from build123d import *

# Parameters (mm, degrees)
SKIZZE2_W                       = 56.2
SKIZZE2_H                       = 56.2
SKIZZE2_W_2                     = 42.2
SKIZZE2_H_2                     = 42.2
AUFSATZ_LINEAR_AUSTRAGEN1_DEPTH = 10
SKIZZE3_W                       = 10
SKIZZE3_H                       = 20
AUFSATZ_LINEAR_AUSTRAGEN2_DEPTH = 20
SKIZZE4_R                       = 2.5
SCHNITT_LINEAR_AUSTRAGEN1_DEPTH = 27
KREISMUSTER1_COUNT              = 3
KREISMUSTER2_COUNT              = 3
VERRUNDUNG1_R                   = 10
VERRUNDUNG2_R                   = 10
VERRUNDUNG3_R                   = 10
VERRUNDUNG4_R                   = 5


with BuildPart() as part:
    # Skizze2 → Aufsatz-Linear austragen1 (new body)
    with BuildSketch(Plane.XY):
        with Locations((21.1, 21.1)):
            Rectangle(SKIZZE2_W, SKIZZE2_H)
        with Locations((21.1, 21.1)):
            Rectangle(SKIZZE2_W_2, SKIZZE2_H_2, mode=Mode.SUBTRACT)
    extrude(amount=AUFSATZ_LINEAR_AUSTRAGEN1_DEPTH)

    # Skizze3 → Aufsatz-Linear austragen2 (add)
    with BuildSketch(Plane(origin=(49.2, 0, 0), x_dir=(0, 0, -1), z_dir=(1, 0, 0))):
        with Locations((-5, 21.1)):
            Rectangle(SKIZZE3_W, SKIZZE3_H)
    aufsatz_linear_austragen2 = extrude(amount=AUFSATZ_LINEAR_AUSTRAGEN2_DEPTH)

    # Skizze4 → Schnitt-Linear austragen1 (cut)
    with BuildSketch(Plane.XY.offset(10)):
        with Locations((59.7, 21.1)):
            Circle(SKIZZE4_R)
    schnitt_linear_austragen1 = extrude(amount=-SCHNITT_LINEAR_AUSTRAGEN1_DEPTH, mode=Mode.SUBTRACT)

    # Kreismuster1: Aufsatz-Linear austragen2 ×3 about axis
    kreismuster1_axis = Axis((21.1, 21.1, 0), (0, 0, 1))
    for i in range(1, KREISMUSTER1_COUNT):
        add(aufsatz_linear_austragen2.rotate(kreismuster1_axis, i * 360 / KREISMUSTER1_COUNT))

    # Kreismuster2: Schnitt-Linear austragen1 ×3 about axis
    kreismuster2_axis = Axis((21.1, 21.1, 0), (0, 0, 1))
    for i in range(1, KREISMUSTER2_COUNT):
        add(schnitt_linear_austragen1.rotate(kreismuster2_axis, i * 360 / KREISMUSTER2_COUNT), mode=Mode.SUBTRACT)

    # Verrundung1
    # the kernel refuses this fillet: 10 mm, written as the material it adds along each edge
    with BuildSketch(Plane(origin=(13.570627693, 49.2, 10), x_dir=(0.866025403783509, 0.5000000000016102, 0), z_dir=(0, 0, -1))) as verrundung1_piece_1:
        with BuildLine():
            CenterArc((11.022527997, -5.183145878), VERRUNDUNG1_R, 120, 28.780734866)
            Line((6.022527997, 3.47710816), (0, 0))
            Line((0, 0), (2.470627693, 0))
        make_face()
    extrude(amount=10)

    # Verrundung2
    # the kernel refuses this fillet: 10 mm, written as the material it takes off along each edge
    with BuildSketch(Plane(origin=(-7, 49.2, -6.36420772), x_dir=(0, -1, 0), z_dir=(0, 0, 1))) as verrundung2_piece_1:
        with BuildLine():
            CenterArc((2.545683088, 10), VERRUNDUNG2_R, 255.251993066, 14.748006934)
            Line((0, 0.329452052), (-0.050913662, 0.136041093))
            ThreePointArc((-0.050913662, 0.136041093), (-0.2, 0.164726026), (-0.2, 0))
            Line((-0.2, 0), (0, -0.2))
            Line((0, -0.2), (2.545683088, -0.2))
            Line((2.545683088, -0.2), (2.545683088, 0))
        make_face()
    extrude(amount=22.72841544, mode=Mode.SUBTRACT)

    # Verrundung3
    # the kernel refuses this fillet: 10 mm, written as the material it adds along each edge
    with BuildSketch(Plane(origin=(13.570627693, -7, 0), x_dir=(1, 0, 0), z_dir=(0, 0, 1))) as verrundung3_piece_1:
        with BuildLine():
            CenterArc((6.95421632, -10), VERRUNDUNG3_R, 90, 28.780734866)
            Line((2.139626345, -1.235313846), (0, 0))
            Line((0, 0), (6.95421632, 0))
        make_face()
    extrude(amount=10)
    # the kernel refuses this fillet: 10 mm, written as the material it takes off along each edge
    with BuildSketch(Plane(origin=(-7, -7, -6.36420772), x_dir=(1, 0, 0), z_dir=(0, 0, 1))) as verrundung3_2_piece_1:
        with BuildLine():
            CenterArc((10, 2.545683088), VERRUNDUNG3_R, 180, 14.748006934)
            Line((0, 2.545683088), (0, 0))
            Line((0, 0), (0.329452052, 0))
        make_face()
    extrude(amount=22.72841544, mode=Mode.SUBTRACT)

    # Verrundung4
    verrundung4_edges = [part.edges().sort_by_distance(p)[0] for p in [
        (49.2, 11.1, 5),
        (49.2, 31.1, 5),
    ]]
    fillet(verrundung4_edges, radius=VERRUNDUNG4_R)


solid = part.part
The model under review builds one solid part; all positions refer to its coordinate system, in mm. A direction names the side the tool comes from. Round coordinates to 2 decimals unless told otherwise and drop trailing zeros. Write each loop counter-clockwise with the first axis right and the second up, starting at its lowest first coordinate (ties: lowest second). Pieces come first, ordered by that corner, then holes. Notation, with made-up numbers: M -22,-14 L 10,-14 A28 cw 10,16 Z; hole C 56,32.25 d2. An arc over 180 degrees is marked long. Use a Markdown table: item, result. Add a question column.
Q1. Insertion check: pin 1 (5 mm diameter, centred on x = 37.5, z = 7.5, fed in from -Y); pin 2 (3 mm diameter, centred on x = 14, z = 2.5, fed in from +Y); pin 3 (4 mm diameter, centred on y = -7, z = 1.5, fed in from +X). Each pin has a flat end and moves straight along its axis. Give the tip position at first contact, or say it passes through.
Q2. To check wall thickness, follow line 1 (X direction, y = 17, z = 9.25); line 2 (Y direction, x = 59.7, z = 7.25); line 3 (Y direction, x = 22.5, z = 1.5). State the ranges of each line that lie inside material, in increasing order.
Q3. We need section A-A, the plane y = 21.1. State the section outline as (x, z) points, plus the area to 3 significant figures.
Q4. We need section D-D, the plane z = 1.25. Count the separate pieces of the cut face and the enclosed holes in it, plus the area to 3 significant figures.
Q5. We need section B-B, the plane x = 33. State the section outline as (y, z) points, plus the area to 3 significant figures.
Q6. We need section C-C, the plane y = 8.5. State the section outline as (x, z) points, plus the area to 3 significant figures.
Q7. The part is to be moulded in two halves that separate along Y. For faces 5 (the face through (-9.106, 53.418, 5.07)), 6 (the face through (-1, 18, 10)), 7 (the face through (62, 11.1, 5)), say which applies: pulls with the +Y half, pulls with the -Y half, needs draft (parallel to the pull), parting line crosses it, or undercut.
Q8. Machinability: for faces 1 (the face through (42.2, 21, 5)), 2 (the face through (49.2, 43, 5)), 3 (the face through (35, -7, 5)), 4 (the face through (-6.92, -5.72, 4.93)), which of the approach directions +Z, -Z, +X, -X, +Y, -Y give a long, thin tool a straight path to every point of the face, cutting with its end or side? Answer none if there is none.
Findings below:
| question | item | result |
|---|---|---|
| 1 | pin 1 | stops at y = -7 |
| 1 | pin 2 | stops at y = 56 |
| 1 | pin 3 | stops at x = 49.2 |
| 2 | line 1 | x = -7 to 0, 42.2 to 69.2 |
| 2 | line 2 | y = 11.1 to 18.6, 23.6 to 31.1 |
| 2 | line 3 | y = -7 to 0, 42.2 to 49.2 |
| 3 | outline | M -7,0 L 0,0 L 0,10 L -7,10 Z; M 42.2,0 L 57.2,0 L 57.2,10 L 42.2,10 Z; M 62.2,0 L 69.2,0 L 69.2,10 L 62.2,10 Z |
| 3 | area | 290 mm² |
| 4 | separate pieces | 1 |
| 4 | enclosed holes | 4 |
| 4 | area | 2,360 mm² |
| 5 | outline | M -7,0 L 0,0 L 0,10 L -7,10 Z; M 42.2,0 L 49.2,0 L 49.2,10 L 42.2,10 Z |
| 5 | area | 140 mm² |
| 6 | outline | M -7,0 L 0,0 L 0,10 L -7,10 Z; M 42.2,0 L 49.81,0 L 49.81,10 L 42.2,10 Z |
| 6 | area | 146 mm² |
| 7 | face 5 | undercut |
| 7 | face 6 | needs draft |
| 7 | face 7 | pulls with the -Y half |
| 8 | face 1 | +Z, -Z |
| 8 | face 2 | +Z, -Z, +X, +Y |
| 8 | face 3 | +Z, -Z, +X, -Y |
| 8 | face 4 | +Z, -Z, -X |
